Input: part model. Units: mm. Frame: model coordinates. Face numbers are marked on the shaded views. A direction names the side the tool comes from. Round coordinates to 2 decimals unless told otherwise and drop trailing zeros. Write each loop counter-clockwise with the first axis right and the second up, starting at its lowest first coordinate (ties: lowest second). Pieces come first, ordered by that corner, then holes. Notation, with made-up numbers: (64, 20) -> (88, 20) arc R33 ccw to (88, 56) -> close; hole circle Ø6 at (63, -15.75). An arc over 180 degrees is marked (long way). Write item = value, one per line.
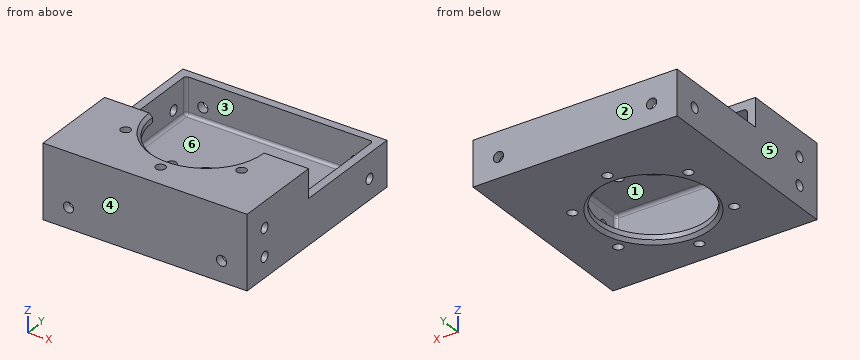
```python
from build123d import *

# Parameters (mm, degrees)
BASE_EXTRUDE_DEPTH = 50.8
SHELL1_T           = -2.032
SKETCH7_R          = 13.5001
CUT_EXTRUDE1_DEPTH = 75.133197314
SKETCH8_R          = 1.27
CUT_EXTRUDE2_DEPTH = 75.133197314
SKETCH9_R          = 1.27
CUT_EXTRUDE3_DEPTH = 75.133197314
SKETCH10_R         = 1.190625
CUT_EXTRUDE4_DEPTH = 75.133197314
CIRPATTERN1_COUNT  = 6
FILLET1_R          = 0.79375
FILLET2_R          = 0.79375
CHAMFER1_SIZE      = 0.79375


with BuildPart() as part:
    # Sketch6 → Base-Extrude (new body)
    with BuildSketch(Plane(origin=(0, 59.342935223, 0), x_dir=(0, 0, -1), z_dir=(1, 0, 0))):
        Polygon((7.112, -8.542935223), (18.288, -8.542935223), (18.288, -59.342935223), (0, -59.342935223), (0, -36.990935223), (7.112, -36.990935223), align=None)
    extrude(amount=-BASE_EXTRUDE_DEPTH)

    # Shell1
    shell1_openings = [part.faces().sort_by_distance(p)[0] for p in [
        (-25.4, 22.352, -3.556),
        (-25.4, 36.576, -7.112),
    ]]
    offset(amount=SHELL1_T, openings=shell1_openings, kind=Kind.INTERSECTION)

    # Sketch7 → Cut-Extrude1 (cut, through all)
    with BuildSketch(Plane.XY):
        with Locations((-25.4, 22.352)):
            Circle(SKETCH7_R)
    extrude(amount=-CUT_EXTRUDE1_DEPTH, mode=Mode.SUBTRACT)

    # Sketch8 → Cut-Extrude2 (cut, through all)
    with BuildSketch(Plane(origin=(0, 0, 0), x_dir=(0, 0, -1), z_dir=(1, 0, 0))):
        with Locations((13.208, 44.45)):
            Circle(SKETCH8_R)
        with Locations((13.208, 6.35)):
            Circle(SKETCH8_R)
        with Locations((6.35, 6.35)):
            Circle(SKETCH8_R)
    extrude(amount=-CUT_EXTRUDE2_DEPTH, mode=Mode.SUBTRACT)

    # Sketch9 → Cut-Extrude3 (cut, through all)
    with BuildSketch(Plane(origin=(0, 50.8, 0), x_dir=(-1, 0, 0), z_dir=(0, 1, 0))):
        with Locations(Location((44.45, -13.208, 0), (0, 0, 90))):
            Circle(SKETCH9_R)
        with Locations(Location((6.35, -13.208, 0), (0, 0, 90))):
            Circle(SKETCH9_R)
    extrude(amount=-CUT_EXTRUDE3_DEPTH, mode=Mode.SUBTRACT)

    # Sketch10 → Cut-Extrude4 (cut, through all)
    with BuildSketch(Plane(origin=(0, 0, -18.288), x_dir=(-1, 0, 0), z_dir=(0, 0, -1))):
        with Locations((25.4, 5.68325)):
            Circle(SKETCH10_R)
    cut_extrude4 = extrude(amount=-CUT_EXTRUDE4_DEPTH, mode=Mode.SUBTRACT)

    # CirPattern1: Cut-Extrude4 ×6 about axis
    cirpattern1_axis = Axis((-25.4, 22.352, 0), (0, 0, 1))
    for i in range(1, CIRPATTERN1_COUNT):
        add(cut_extrude4.rotate(cirpattern1_axis, i * 360 / CIRPATTERN1_COUNT), mode=Mode.SUBTRACT)

    # Fillet1
    fillet1_edges = [part.edges().sort_by_distance(p)[0] for p in [
        (-48.768, 25.4, -16.256),
        (-48.768, 12.192, -2.032),
        (-2.032, 12.192, -2.032),
        (-2.032, 25.4, -16.256),
    ]]
    fillet(fillet1_edges, radius=FILLET1_R)

    # Fillet2
    fillet2_edges = [part.edges().sort_by_distance(p)[0] for p in [
        (-48.768, 2.032, -9.144),
        (-48.768, 48.768, -11.287125),
        (-2.032, 48.768, -11.287125),
        (-25.4, 48.768, -16.256),
        (-2.264483992, 48.768, -16.023516008),
        (-48.535516008, 48.768, -16.023516008),
        (-25.4, 2.032, -16.256),
        (-2.032, 2.032, -9.144),
        (-25.4, 2.032, -2.032),
        (-48.535516008, 2.032, -2.264483992),
        (-2.264483992, 2.032, -2.264483992),
        (-2.264483992, 2.032, -16.023516008),
        (-48.535516008, 2.032, -16.023516008),
    ]]
    fillet(fillet2_edges, radius=FILLET2_R)

    # Chamfer1
    chamfer1_edges = [part.edges().sort_by_distance(p)[0] for p in [
        (-38.9001, 22.352, -18.288),
        (-25.4, 8.8519, 0),
    ]]
    chamfer(chamfer1_edges, length=CHAMFER1_SIZE)


solid = part.part
```
1) Draft query along Y for the marked faces 1, 2, 3 and 4. Return one class per face: +Y half, -Y half, draft (parallel to the pull), parting line (faces both ways), or undercut.
Solutions:
face_1 = draft
face_2 = +Y half
face_3 = undercut
face_4 = -Y half
2) Line query: L1, parallel to X at y = 29, z = -10.75; L2, parallel to Y at x = -36, z = -10.75; L3, parallel to Z at x = -10, y = 21.5. Output: solid intervals per line, ascending. Write a range as from..to.
Solutions:
L1 = -50.8..-48.77, -2.03..0
L2 = 0..2.03, 48.77..50.8
L3 = -18.29..-16.26, -2.03..0
3) Cut plane D-D (x = -44.45). Return the cut outline in (y, z).
Solutions:
outline = (0, -18.29) -> (50.8, -18.29) -> (50.8, -14.48) -> (48.77, -14.48) -> (48.77, -15.46) arc R0.79 cw to (47.97, -16.26) -> (2.83, -16.26) arc R0.79 cw to (2.03, -15.46) -> (2.03, -14.48) -> (0, -14.48) -> close; (0, -11.94) -> (2.03, -11.94) -> (2.03, -2.83) arc R0.79 cw to (2.83, -2.03) -> (22.35, -2.03) -> (22.35, 0) -> (0, 0) -> close; (48.77, -11.94) -> (50.8, -11.94) -> (50.8, -7.11) -> (48.77, -7.11) -> close
4) Cut plane B-B (z = -10.75). Return the cut outline in (x, y), and give its area (3 significant figures).
Solutions:
outline = (-50.8, 0) -> (0, 0) -> (0, 50.8) -> (-50.8, 50.8) -> close; hole (-48.77, 2.83) arc R0.79 ccw to (-47.97, 2.03) -> (-2.83, 2.03) arc R0.79 ccw to (-2.03, 2.83) -> (-2.03, 47.97) arc R0.79 ccw to (-2.83, 48.77) -> (-47.97, 48.77) arc R0.79 ccw to (-48.77, 47.97) -> close
area = 397 mm^2
5) Access query for the marked faces 5 and 6. Directions: +Z, -Z, +X, -X, +Y, -Y. A direction counts if a zero-diameter tool reaches every point of the face in a straight line with its end or side. Return the directions, or none.
Solutions:
face_5 = +Z, -Z, -X, +Y, -Y
face_6 = none
6) Cut plane C-C (z = -6.35). Return the cut outline in (x, y).
Solutions:
outline = (-50.8, 0) -> (0, 0) -> (0, 5.08) -> (-2.03, 5.08) -> (-2.03, 2.83) arc R0.79 cw to (-2.83, 2.03) -> (-47.97, 2.03) arc R0.79 cw to (-48.77, 2.83) -> (-48.77, 5.08) -> (-50.8, 5.08) -> close; (-50.8, 7.62) -> (-48.77, 7.62) -> (-48.77, 22.35) -> (-50.8, 22.35) -> close; (-2.03, 7.62) -> (0, 7.62) -> (0, 22.35) -> (-2.03, 22.35) -> close
7) First-contact query: P1, Ø14, axis at x = -37, y = 39, coming from the +Z side; P2, Ø3.5, axis at x = -46.5, z = -3, coming from the +Y side; P3, Ø1.5, axis at x = -34.5, z = -5, coming from the +Y side; P4, Ø1.5, axis at x = -44.45, z = -13.208, coming from the +Y side. Flat tips, straight axial feed; report the tip coordinate or a pass-through.
Solutions:
P1 = -16.26
P2 = 22.35
P3 = 2.03
P4 = through
8) Cut plane A-A (x = -25.4). Count the separate pieces of the cut face and the enclosed holes in it, and give its area (3 significant figures).
Solutions:
separate_pieces = 5
enclosed_holes = 0
area = 98.8 mm^2
